The listing builds one solid part. Answer for the finished solid, in the listing's coordinates (mm). Round coordinates to 2 decimals unless told otherwise and drop trailing zeros. Write each loop counter-clockwise with the first axis right and the second up, starting at its lowest first coordinate (ties: lowest second). Pieces come first, ordered by that corner, then holes.
Item 1: For a pull along Y with two mould halves and no side action, classify faces 1 (the face through (0.06, 11.52, 1.66)), 2 (the face through (0, 62.1, 0)), 3 (the face through (-3.905, 30.615, -0.867)) as +Y half, -Y half, draft (parallel to the pull), parting line (faces both ways), or undercut.
Item 2: Find the intervals of material crossed by probe 1 along Y at (x, z) = (-0.5, 0); probe 2 along Y at (x, z) = (-1.75, -1.5); probe 3 along Z at (x, y) = (-2.5, 46.5), in increasing order.
Item 3: Find section D-D on y = 10. Give the vertices of the cut face in (x, z), then the cut area to 3 significant figures.
Item 4: Find section B-B on x = 0. Give the vertices of the cut face in (y, z).
Item 5: Find section C-C on y = 33. Give the vertices of the cut face in (x, z), then the cut area to 3 significant figures.
Item 6: This flat-tipped pin is pushed along its axis until it touches: pin 1 (4 mm diameter, centred on x = 2, z = -0.5, fed in from -Y). Where does it stop, or does it pass through?
Item 7: Find section A-A on z = 0. Give the vertices of the cut face in (x, y).
```python
from build123d import *

# Parameters (mm, degrees)
SKETCH1_R            = 4
BOSS_EXTRUDE1_DEPTH  = 62.1
M5_CLEARANCE_HOLE1_D = 5.5
M4_CLEARANCE_HOLE1_D = 4.5


with BuildPart() as part:
    # Sketch1 → Boss-Extrude1 (new body)
    with BuildSketch(Plane(origin=(0, 0, 0), x_dir=(1, 0, 0), z_dir=(0, 1, 0))):
        with Locations(Location((0, 0, 0), (0, 0, 270))):
            Circle(SKETCH1_R)
    extrude(amount=BOSS_EXTRUDE1_DEPTH)

    # M5 Clearance Hole1 (through all)
    with Locations(Plane(origin=(-4, 0, 0), x_dir=(0, 0, -1), z_dir=(-1, 0, 0))):
        with Locations((0, -47.1)):
            Hole(M5_CLEARANCE_HOLE1_D / 2)

    # M4 Clearance Hole1 (through all)
    with Locations(Plane.ZY.offset(4)):
        with Locations((0, 10)):
            Hole(M4_CLEARANCE_HOLE1_D / 2)


solid = part.part
```
Check values:
1. face 1: undercut
1. face 2: +Y half
1. face 3: draft
2. probe 1: y = 0 to 7.75, 12.25 to 44.35, 49.85 to 62.1
2. probe 2: y = 0 to 8.32, 11.68 to 44.8, 49.4 to 62.1
2. probe 3: z = -3.12 to -2.68, 2.68 to 3.12
3. outline: (-3.31, -2.25) arc R4 ccw to (3.31, -2.25) - close; (-3.31, 2.25) - (3.31, 2.25) arc R4 ccw to start
3. area: 16.3 mm2
4. outline: (0, -4) - (62.1, -4) - (62.1, 4) - (0, 4) - close; hole circle Ø4.5 at (10, 0); hole circle Ø5.5 at (47.1, 0)
5. outline: circle Ø8 at (0, 0)
5. area: 50.3 mm2
6. pin 1: stops at y = 0
7. outline: (-4, 0) - (4, 0) - (4, 7.75) - (-4, 7.75) - close; (-4, 12.25) - (4, 12.25) - (4, 44.35) - (-4, 44.35) - close; (-4, 49.85) - (4, 49.85) - (4, 62.1) - (-4, 62.1) - close
